Source: CAD feature listing. Evaluate the final solid. Frame: model axes, mm. A direction names the side the tool comes from. Give positions to 0.01 mm unless a question says otherwise; leave off trailing zeros. Order: outer loops, then holes, each group sorted by start corner. A loop starts at its lowest first (then second) coordinate and runs counter-clockwise, first axis right, second up. Notation, with made-up numbers: M -22,43.5 L -12,43.5 A31 ccw -12,79.5 Z; hole C -26,62.25 d4. An arc over 180 degrees is marked long. Answer as a JSON object with one key per item and string values. Group by question number.
1. Section query A-A (x = 60). Output: boundary loops of the cut face in (y, z) (3 decimals).
2. Set-up query: faces 1 (the flat face through (-19.05, 53, 75)), 2 (the flat face through (-2, -24, 44.45)), 3 (the flat face through (-2, -114.3, 32)). Return all of +Z, -Z, +X, -X, +Y, -Y with unobstructed straight access to the full face (end or side cutting, diameter ignored); none if empty.
3. Section query D-D (x = -180.5). Output: boundary loops of the cut face in (y, z) (3 decimals), plus the area to 3 significant figures.
4. Pin query (flat end, axial travel): P1, Ø1.9, axis at x = -88, y = -24, coming from the -Z side; P2, Ø9.5, axis at y = 74, z = 7.5, coming from the -X side; P3, Ø1, axis at y = 18.5, z = 432.5, coming from the +X side; P4, Ø2, axis at x = 153.5, z = 982, coming from the -Y side (3 decimals). Return the tip coordinate at first contact, or that it passes through.
5. Section query B-B (z = 990). Output: boundary loops of the cut face in (x, y) (3 decimals), plus the area to 3 significant figures.
6. Section query C-C (y = -90). Output: boundary loops of the cut face in (x, z), plus the area to 3 significant figures.
7. Material intervals for L1, parallel to Y at x = -11.5, z = 987.5 (3 decimals); L2, parallel to Z at x = -25.5, y = 122.5; L3, parallel to Y at x = -152.5, z = 1062.5 (3 decimals), sorted ascending. Write a range as [from, to].
from build123d import *

# Parameters (mm, degrees)
F0_W      = 304.8
F0_H      = 304.8
F1_DEPTH  = 19.05
F2_W      = 228.6
F2_H      = 228.6
F3_DEPTH  = 25.4
F4_W      = 88.9
F4_H      = 44.45
F5_DEPTH  = 1219.2
F6_W      = 38.1
F6_H      = 79.375
F7_DEPTH  = 80.01
F9_DEPTH  = 50.8
F10_W     = 508
F10_H     = 254
F11_DEPTH = 6.35


with BuildPart() as f1:
    # F0 (on Top) → F1 (new body)
    with BuildSketch(Plane.XY):
        Rectangle(F0_W, F0_H)
    extrude(amount=F1_DEPTH)

    # F2 (on face) → F3 (join)
    with BuildSketch(Plane.XY.offset(19.05)):
        Rectangle(F2_W, F2_H)
    extrude(amount=F3_DEPTH)

    # F4 (on face) → F5 (join)
    with BuildSketch(Plane.XY.offset(44.45)):
        Rectangle(F4_W, F4_H)
    extrude(amount=F5_DEPTH)

    # F6 (on face) → F7 (join)
    with BuildSketch(Plane.XY.offset(44.45)):
        with Locations((0, 61.9125)):
            Rectangle(F6_W, F6_H)
    extrude(amount=F7_DEPTH)

    # F8 (on face) → F9 (cut)
    with BuildSketch(Plane(origin=(-19.05, 0, 0), x_dir=(0, -1, 0), z_dir=(-1, 0, 0))):
        Polygon((-101.6, 124.46), (-101.6, 44.45), (-22.225, 124.46), align=None)
    extrude(amount=-F9_DEPTH, mode=Mode.SUBTRACT)

    # F10 (on face) → F11 (join)
    with BuildSketch(Plane.XZ.offset(22.225)):
        with Locations((0, 1060.45)):
            Rectangle(F10_W, F10_H)
    extrude(amount=F11_DEPTH)


solid = f1.part
Answer sheet:
{
 "1": {"outline": "M -152.4,0 L 152.4,0 L 152.4,19.05 L 114.3,19.05 L 114.3,44.45 L -114.3,44.45 L -114.3,19.05 L -152.4,19.05 Z; M -28.575,933.45 L -22.225,933.45 L -22.225,1187.45 L -28.575,1187.45 Z"},
 "2": {"face 1": "+Z, -X, +Y", "face 2": "none", "face 3": "+Z, +X, -X, -Y"},
 "3": {"outline": "M -28.575,933.45 L -22.225,933.45 L -22.225,1187.45 L -28.575,1187.45 Z", "area": "1,610 mm^2"},
 "4": {"P1": "z = 0", "P2": "x = -152.4", "P3": "x = 44.45", "P4": "y = -28.575"},
 "5": {"outline": "M -254,-28.575 L 254,-28.575 L 254,-22.225 L 44.45,-22.225 L 44.45,22.225 L -44.45,22.225 L -44.45,-22.225 L -254,-22.225 Z", "area": "7,180 mm^2"},
 "6": {"outline": "M -152.4,0 L 152.4,0 L 152.4,19.05 L 114.3,19.05 L 114.3,44.45 L -114.3,44.45 L -114.3,19.05 L -152.4,19.05 Z", "area": "11,600 mm^2"},
 "7": {"L1": "[-28.575, 22.225]", "L2": "[0, 19.05]", "L3": "[-28.575, -22.225]"}
}
